Could you check a few things on this model? Use its own coordinates, in mm. A direction names the side the tool comes from. Give positions to 0.01 mm unless a question says otherwise; leave off trailing zeros. Order: outer loops, then holes, each group sorted by start corner. A loop starts at its lowest first (then second) coordinate and runs counter-clockwise, first axis right, second up.
Autodesk Inventor part; units mm, degrees
ref_plane "YZ Plane" through (0, 0, 0) normal (1, 0, 0) x (0, 1, 0)
ref_plane "XZ Plane" through (0, 0, 0) normal (0, 1, 0) x (-1, 0, 0)
ref_plane "XY Plane" through (0, 0, 0) normal (0, 0, 1) x (1, 0, 0)
sketch "スケッチ1" plane through (0, 0, 0) normal (0, 1, 0) x (-1, 0, 0)
  circle A0 centre (0, 0) radius 1.15
  circle A1 centre (0, 0) radius 2
  circle A2 centre (0, 0) radius 2.9
  line L0 (-2, 0) -> (2, 0)
  line L1 (2, 0) -> (2, -2.9)
  line L2 (2, -2.9) -> (-2, -2.9)
  line L3 (-2, -2.9) -> (-2, 0)
  line L4 (0, 0) -> (0, 2.9)
  line L5 (0, 0) -> (2.9, 0)
  line L6 (2.9, 0) -> (2.9, 10)
  line L7 (2.9, 10) -> (0, 10)
  line L8 (0, 10) -> (0, 0)
  point P0 (0, 2)
  point P1 (2, -2.1)
  point P2 (-2, -2.1)
  dimension "d1" = 4
  dimension "d2" = 5.8
  dimension "d0" = 2.3
  dimension "d3" = 10
extrude "押し出し1" add sketch "スケッチ1" along normal blind 4.5 contours L5 A2 L1 | A1 L4 A2 L5 | A2 L8 L7 L6
extrude "押し出し2" add sketch "スケッチ1" along normal blind 3.5 contours A1 L3 A2 L4
extrude "押し出し3" add sketch "スケッチ1" against normal blind 1 contours L0 A1 A0 | A0 L4 A1 L0 | A0 L0 A1 L4 | L1 A2 L3 A1 | L5 A2 L1 | A1 L4 A2 L5 | A1 L3 A2 L4 | A2 L8 L7 L6
sketch "スケッチ2" plane through (-2.9, 4.5, 10) normal (0, 0, 1) x (1, 0, 0)
  line L0 (2.9, -4.5) -> (1.4, -4.5)
  line L1 (1.4, -4.5) -> (1.4, -4)
  line L2 (1.4, -4) -> (2.9, -4)
  line L3 (2.9, -4) -> (2.9, -4.5)
  dimension "d10" = 1.5
  dimension "d11" = 0.5
hole "穴1" at (-1.5, 0.5, 10) direction (0, 0, -1) diameter 1 end through all
sketch "スケッチ3" plane through (-2.9, 4.5, 10) normal (0, 0, 1) x (1, 0, 0)
  line L0 (0.9, 0) -> (0, 0)
  line L1 (0, 0) -> (4, 0)
  line L2 (4, 0) -> (4, -4)
  line L3 (4, -4) -> (0, -4)
  line L4 (0, -4) -> (0, 0)
  line L5 (0, 0) -> (3.25, 0)
  line L6 (3.25, 0) -> (3.25, -3.25)
  line L7 (3.25, -3.25) -> (0, -3.25)
  line L8 (0, -3.25) -> (0, 0)
  line L9 (0, 0) -> (1.625, 0)
  line L10 (1.625, 0) -> (1.625, -1.625)
  line L11 (1.625, -1.625) -> (0, -1.625)
  line L12 (0, -1.625) -> (0, 0)
  point P0 (2.9, -4.5)
  dimension "d19" = 4
  dimension "d20" = 4
  dimension "d21" = 3.25
  dimension "d22" = 3.25
extrude "押し出し4" add sketch "スケッチ3" along normal blind 10 and the other way blind 3 contours L1 L10 L11 L4 L0 | L1 L6 L7 L4 L11 L10
fillet "フィレット1" radius 2 1 edges at (0.35, 2.875, 7)
sketch "スケッチ4" plane through (-2.9, 4.5, 20) normal (0, 0, 1) x (1, 0, 0)
  line L0 (0.9, 0) -> (0, 0)
  line L1 (0, 0) -> (1.625, 0)
  line L2 (1.625, 0) -> (1.625, -1.625)
  line L3 (1.625, -1.625) -> (0, -1.625)
  line L4 (0, -1.625) -> (0, 0)
  circle A0 centre (1.625, -1.625) radius 1.05
  point P0 (2.9, -4.5)
  dimension "d28" = 1.625
  dimension "d29" = 1.625
  dimension "d30" = 2.1
extrude "押し出し5" cut sketch "スケッチ4" against normal blind 11 contours A0 L3 L2 | L2 L3 A0
properties part number "srod1.5right"
Item 1: For pin 1 (2.5 mm diameter, centred on x = 0, z = 0, fed in from +Y); pin 2 (0.7 mm diameter, centred on x = -2, y = 0.5, fed in from +Z); pin 3 (1.5 mm diameter, centred on x = 0.5, y = 1.5, fed in from -Z), each with a flat end and sliding along its axis, tell me the tip position at first contact or that it passes through.
Findings:
pin 1: stops at y = 0
pin 2: stops at z = 10
pin 3: stops at z = 1.56
Item 2: Please list where these lines run through material, in increasing order: line 1 along X through (y, z) = (-0.4, 0); line 2 along X through (y, z) = (0.55, 3); line 3 along Y through (x, z) = (-1.5, 4.75).
Findings:
line 1: x = -2.9 to -1.15, 1.15 to 2.9
line 2: x = -2.9 to -2, -1 to 0
line 3: y = -1 to 0, 1 to 4.5
Item 3: Imagine slicing it at C-C on y = 1.45. List the corners of the cut face in (x, z) for me, then the cut area to 3 significant figures.
Findings:
outline: (-2.9, 0) arc R2.9 ccw to (-2, -2.1) - (-2, 0) arc R2 cw to (2, 0) - (2, -2.1) arc R2.9 ccw to (0, 2.9) - (0, 7) arc R2 ccw to (0.35, 8.13) - (0.35, 20) - (-2.9, 20) - close
area: 65.4 mm2
Item 4: For faces 4 (the flat face through (0, 0, -2)), 5 (the cylindrical face through (-2.049, 3.585, 14.577)), 6 (the cylindrical face through (0.263, 2.898, 7.547)), which set-ups out of +Z, -Z, +X, -X, +Y, -Y let a thin tool reach every point of the face, with its end or its side?
Findings:
face 4: -Z, +Y
face 5: +Z
face 6: +X, +Y, -Y
Item 5: Imagine slicing it at B-B on z = 3.5. List the corners of the cut face in (x, y) for me.
Findings:
outline: (-2.9, -1) - (0, -1) - (0, 4.5) - (-2.9, 4.5) - close; hole circle Ø1 at (-1.5, 0.5)
Item 6: Imagine slicing it at A-A on y = -0.55. List the corners of the cut face in (x, z) for me, then the cut area to 3 significant figures.
Findings:
outline: (-2.9, 0) arc R2.9 ccw (long way) to (0, 2.9) - (0, 10) - (-2.9, 10) - close; hole circle Ø2.3 at (0, 0)
area: 44.7 mm2
Item 7: Imagine slicing it at D-D on x = 1.35. List the corners of the cut face in (y, z) for me, then the cut area to 3 significant figures.
Findings:
outline: (-1, -2.57) - (0, -2.57) - (0, 1.48) - (3.5, 1.48) - (3.5, 2.57) - (-1, 2.57) - close
area: 8.95 mm2
Item 8: We'd pull the mould along Z, two halves only. Please class faces 1 (the flat face through (-1, 0, 10)), 2 (the cylindrical face through (0.91, -0.49, -0.7)), 3 (the flat face through (0.35, 3, 14)): +Z half, -Z half, draft (parallel to the pull), parting line (faces both ways), or undercut.
Findings:
face 1: +Z half
face 2: undercut
face 3: draft
